Model file for the job. Use its own axes, mm. A direction names the side the tool comes from. Give positions to 0.01 mm unless a question says otherwise; leave off trailing zeros. Answer in a Markdown table with one row per item. Add a question column.
Autodesk Inventor part; units mm, degrees
ref_plane "Work Plane1" through (0, 0, 0) normal (0.6427876, -0.7660444, 0) x (0, 0, -1)
ref_plane "Work Plane2" through (0, 14.3, -20) normal (-0.6427876, 0.7660444, 0) x (0, 0, -1)
ref_plane "YZ Plane" through (0, 0, 0) normal (1, 0, 0) x (0, 1, 0)
sketch "Sketch1" plane through (0, 0, 0) normal (0, 1, 0) x (-1, 0, 0)
  circle A0 centre (0, 0) radius 5.075
  circle A1 centre (0, 0) radius 20
  line L0 (1.5, -3.825) -> (-1.5, -3.825)
  line L1 (-1.5, -3.825) -> (-1.5, -6.325)
  line L2 (-1.5, -6.325) -> (1.5, -6.325)
  line L3 (1.5, -6.325) -> (1.5, -3.825)
  line L4 (1.5, -3.825) -> (-1.5, -6.325) construction
  line L5 (-1.5, -3.825) -> (1.5, -6.325) construction
  circle A2 centre (0, 0) radius 2.5
  circle A3 centre (0, 0) radius 8.754
  point P0 (0, -5.075)
  point P1 (-1.5, -4.8483)
  point P2 (1.5, -4.8483)
  dimension "d0" = 10.15
  dimension "d1" = 40
  dimension "d2" = 1.25
  dimension "d3" = 3
  dimension "d17" = 5
extrude "Extrusion1" add sketch "Sketch1" along normal blind 14.3 contours A1 | A3
sketch "Sketch2" plane through (0, 0, 0) normal (1, 0, 0) x (0, 1, 0)
  line L0 (0, 0) -> (14.3, 0)
  line L1 (14.3, 0) -> (14.3, -20)
  line L2 (14.3, -20) -> (0, -20) construction
  line L3 (0, -20) -> (0, 0)
  line L4 (0, -20) -> (14.3, -20) construction
  line L5 (14.3, -20) -> (14.3, -20.0661)
  line L6 (0, -20) -> (14.3, -20)
  circle A0 centre (7.15, -20) radius 2.5
  line L7 (9.65, -20) -> (4.65, -20)
  line L8 (4.65, -20) -> (4.65, -28)
  line L9 (4.65, -28) -> (9.65, -28)
  line L10 (9.65, -28) -> (9.65, -20)
  line L11 (14.3, -20) -> (0, -20)
  line L12 (0, -20) -> (0, -25)
  line L13 (0, -25) -> (14.3, -25)
  line L14 (14.3, -25) -> (14.3, -20)
  point P0 (4.65, -25)
  point P1 (14.3, -20)
  point P2 (9.65, -25)
  point P3 (14.3, -20)
  point P4 (14.3, -20)
  dimension "d22" = 5
  dimension "d7" = 20
  dimension "d10" = 14.3
  dimension "d23" = 8
  dimension "d31" = 5
  dimension "d41" = 14.3
  dimension "d42" = 5
revolve "Revolution1" add sketch "Sketch2" angle 360 about axis through (0, 0, 0) along (0, 1, 0) contours L6 L8 L13 L12 | L5 L14 L13 L10 L6
extrude "Extrusion3" add sketch "Sketch1" against normal blind 2 contours A0 L3 L0 L1 | L1 L0 L3 A0 | A0 L3 L2 L1 | A3
revolve "Revolution4" cut sketch "Sketch2" angle 360 about axis through (0, 0, 0) along (0, 1, 0) contours A0 L6 | L6 A0
sketch "Sketch3" plane through (0, 0, 0) normal (0, -1, 0) x (1, 0, 0)
  line L0 (0, 0) -> (0, -22)
  dimension "d25" = 22
ref_plane "Work Plane1" through (0, 0, 0) normal (0.6427876, -0.7660444, 0) x (0, 0, -1)
sketch "Sketch4" plane through (0, 0, 0) normal (0.6427876, -0.7660444, 0) x (0, 0, -1)
  ellipse E0 centre (0, 2.7318) end of major axis (22, 2.7318) minor radius 16.853
  line L0 (0, 0) -> (18, 0)
  circle A0 centre (18, 0) radius 2.5
  dimension "d27" = 18
  dimension "d28" = 5
extrude "Extrusion4" cut sketch "Sketch4" against normal blind 9 contours A0
extrude "Extrusion5" cut sketch "Sketch4" along normal blind 7 contours A0
ref_plane "Work Plane2" through (0, 14.3, -20) normal (-0.6427876, 0.7660444, 0) x (0, 0, -1)
sketch "Sketch5" plane through (0, 14.3, -20) normal (-0.6427876, 0.7660444, 0) x (0, 0, -1)
  ellipse E0 centre (-20, 0) end of major axis (-25.075, 0) minor radius 3.8877 (-15.1517, 1.1491) -> (-15.1517, -1.1491) ccw
  line L0 (-20, 0) -> (-2, 0)
  circle A0 centre (-2, 0) radius 2.5
  point P0 (-20, 9.1919)
  dimension "d36" = 5
  dimension "d56" = 18
extrude "Extrusion6" cut sketch "Sketch5" against normal blind 9
extrude "Extrusion7" cut sketch "Sketch5" along normal blind 8
extrude "Extrusion8" cut sketch "Sketch1" along normal through all contours A0 L3 L0 L1 | L1 L0 L3 A0 | A0 L3 L2 L1
sketch "Sketch6" plane through (0, 14.3, 0) normal (0, 1, 0) x (1, 0, 0)
  circle A0 centre (0, 0) radius 15
  circle A1 centre (0, 0) radius 35.6972
  dimension "d45" = 30
extrude "Extrusion9" cut sketch "Sketch6" against normal blind 2.5
sketch "Sketch7" plane through (0, 0, 0) normal (0, -1, 0) x (1, 0, 0)
  circle A0 centre (0, 0) radius 2.5
  circle A1 centre (0, 0) radius 20
  line L0 (24, -7.5) -> (-24, -7.5)
  line L1 (-24, -7.5) -> (-24, 7.5)
  line L2 (-24, 7.5) -> (24, 7.5)
  line L3 (24, 7.5) -> (24, -7.5)
  line L4 (24, -7.5) -> (-24, 7.5) construction
  line L5 (-24, -7.5) -> (24, 7.5) construction
  circle A2 centre (0, 0) radius 11
  circle A3 centre (20, 0) radius 2.175
  circle A4 centre (-20, 0) radius 2.175
  dimension "d48" = 40
  dimension "d49" = 48
  dimension "d50" = 15
  dimension "d51" = 22
  dimension "d52" = 4.35
  dimension "d53" = 4.35
extrude "Extrusion10" cut sketch "Sketch7" against normal blind 4.25 contours A1 A3 | A1 A3 | A4 A1 | A1 A4
fillet "Fillet1" radius 1.5 1 edges at (0, 9.65, 25)
properties part number "spool_temp"
Item 1: Pin check, flat tips, straight feed: pin 1 Ø3.5 at (x, z) = (-20, 0) entering from +Y; pin 2 Ø3.5 at (x, z) = (-20.5, -0.5) entering from -Y; pin 3 Ø0.9 at (x, y) = (0, 10.5) entering from +Z. Stop position of each tip, or through.
Item 2: Two-plate mould, pull along X, no slides. Class faces 6 (the flat face through (-2, -2, -2)), 7 (the cylindrical face through (17.827, 2.095, 0.096)), 8 (the cylindrical face through (-7.509, 2.358, -23.846)): pulls with the +X half, pulls with the -X half, needs draft (parallel to the pull), parting line crosses it, or undercut.
Item 3: Which spindle directions (+Z, -Z, +X, -X, +Y, -Y) get a long thin tool onto all of the face, cutting with end or side? Do faces 1 (the flat face through (17, 9.65, 11)), 2 (the cylindrical face through (-7.509, 11.48, -23.846)), 3 (the flat face through (0, 0, -11)), 4 (the cylindrical face through (-14.985, 13.068, -0.66)), 5 (the flat face through (-5.59, 7.06, -16.24)). Say none if no direction does.
Item 4: Wall check: line 1 (X direction, y = 2.15, z = 0) (3 decimals); line 2 (Y direction, x = 16.5, z = -16); line 3 (Z direction, x = -20, y = 3.15) (3 decimals). Give the ranges that are in metal, low to high.
Evaluation:
| question | item | result |
|---|---|---|
| 1 | pin 1 | stops at y = 11.8 |
| 1 | pin 2 | stops at y = 0 |
| 1 | pin 3 | stops at z = 24.99 |
| 2 | face 6 | needs draft |
| 2 | face 7 | undercut |
| 2 | face 8 | parting line crosses it |
| 3 | face 1 | none |
| 3 | face 2 | +Y, -Y |
| 3 | face 3 | -Y |
| 3 | face 4 | +Y |
| 3 | face 5 | -Z |
| 4 | line 1 | x = -25 to -22.175, -17.825 to -5.075, 5.075 to 17.825, 22.175 to 25 |
| 4 | line 2 | y = 0 to 4.65, 9.65 to 11.8 |
| 4 | line 3 | z = -15 to -2.175, 2.175 to 15 |
